Source: CAD feature listing. Evaluate the final solid. Frame: model axes, mm. A direction names the side the tool comes from. Round coordinates to 2 decimals unless told otherwise and drop trailing zeros. Loops run counter-clockwise (first coordinate to the right, second up) from the corner with the lowest first, then second, coordinate; pieces in that order, holes last. Notation, with made-up numbers: M 15,10 L 58,10 A31 ccw 58,41 Z; hole C -12,41 d9. An arc over 180 degrees is marked long. Answer as a JSON object with one key per item and string values.
Autodesk Inventor part; units mm, degrees
ref_plane "YZ Plane" through (0, 0, 0) normal (1, 0, 0) x (0, 1, 0)
ref_plane "XZ Plane" through (0, 0, 0) normal (0, 1, 0) x (-1, 0, 0)
ref_plane "XY Plane" through (0, 0, 0) normal (0, 0, 1) x (1, 0, 0)
sketch "Sketch1" plane through (0, 0, 0) normal (0, 0, 1) x (-1, 0, 0)
  line L0 (0, -67.1677) -> (0, 491.6323)
  line L1 (0, 491.6323) -> (-95.25, 491.6323)
  line L2 (-95.25, 491.6323) -> (-95.25, 485.2823)
  line L3 (-95.25, 485.2823) -> (-63.5, 485.2823)
  line L4 (-63.5, 485.2823) -> (-60.325, 482.1073)
  line L5 (-60.325, 482.1073) -> (-63.5308, 477.5289)
  line L6 (-63.5308, 477.5289) -> (-76.2, 477.5289)
  line L7 (-76.2, 477.5289) -> (-76.2, 375.9289)
  line L8 (-76.2, 375.9289) -> (-133.35, 375.9289)
  line L9 (-133.35, 375.9289) -> (-133.35, 350.5289)
  line L10 (-133.35, 350.5289) -> (-127, 346.0826)
  line L11 (-127, 346.0826) -> (-127, 25.4)
  line L12 (-127, 25.4) -> (-139.7, 25.4)
  line L13 (-139.7, 25.4) -> (-139.7, 0)
  line L14 (-139.7, 0) -> (0, 0)
  line L15 (0, 0) -> (0, 491.6323)
  dimension "d1" = 127
  dimension "d2" = 25.4
  dimension "d3" = 12.7
  dimension "d4" = 95.25
  dimension "d5" = 6.35
  dimension "d6" = 558.8
  dimension "d7" = 6.35
  dimension "d9" = 63.5
  dimension "d10" = 76.2
  dimension "d11" = 101.6
  dimension "d12" = 35
  dimension "d13" = 135
  dimension "d14" = 25.4
  dimension "d15" = 3.175
revolve "Revolution1" add sketch "Sketch1" angle 360 about axis through (0, 67.1677, 0) along (0, -1, 0)
properties part number "Newport SL 1200-422"
Item 1: Section A-A on z = 0. Return the cut outline in (x, y) (3 decimals), then the cut area to 3 significant figures.
Answer sheet:
{"outline": "M -139.7,-25.4 L -127,-25.4 L -127,-346.083 L -133.35,-350.529 L -133.35,-375.929 L -76.2,-375.929 L -76.2,-477.529 L -63.531,-477.529 L -60.325,-482.107 L -63.5,-485.282 L -95.25,-485.282 L -95.25,-491.632 L 95.25,-491.632 L 95.25,-485.282 L 63.5,-485.282 L 60.325,-482.107 L 63.531,-477.529 L 76.2,-477.529 L 76.2,-375.929 L 133.35,-375.929 L 133.35,-350.529 L 127,-346.083 L 127,-25.4 L 139.7,-25.4 L 139.7,0 L -139.7,0 Z", "area": "114,000 mm²"}
Item 2: Pull-direction query (Y, two-part tool) for faces 1 (the flat face through (17, -477.529, -62)), 2 (the flat face through (-2, 0, 2)), 3 (the flat face through (20, -485.282, -62)), 4 (the flat face through (-1, -491.632, 1)); classes: pulls with the +Y half, pulls with the -Y half, needs draft (parallel to the pull), parting line crosses it, or undercut.
Answer sheet:
{"face 1": "undercut", "face 2": "pulls with the +Y half", "face 3": "undercut", "face 4": "pulls with the -Y half"}
Item 3: Access query for faces 5 (the cylindrical face through (-110.86, -12.52, 85.01)), 6 (the cylindrical face through (-75.587, -488.413, 57.958)), 7 (the flat face through (30, -25.4, -124)). Directions: +Z, -Z, +X, -X, +Y, -Y. A direction counts if a zero-diameter tool reaches every point of the face in a straight line with its end or side. Return the directions, or none.
Answer sheet:
{"face 5": "+Y, -Y", "face 6": "-Y", "face 7": "none"}
Item 4: Contact query for flat-ended pins moving along their axis: pin 1 Ø2 at (x, y) = (-14.5, -423.5) entering from +Z; pin 2 Ø5 at (x, y) = (-9, -250.5) entering from -Z; pin 3 Ø10 at (x, y) = (-60, -133) entering from -Z. Output: stop coordinate, or through.
Answer sheet:
{"pin 1": "stops at z = 74.99", "pin 2": "stops at z = -126.83", "pin 3": "stops at z = -114.47"}
Item 5: Line query: probe 1 along Y at (x, z) = (-84, 37.5); probe 2 along Y at (x, z) = (44, -116.5); probe 3 along X at (y, z) = (-422.5, -1). Output: solid intervals per line, ascending. Write a range as from..to.
Answer sheet:
{"probe 1": "y = -491.63..-485.28, -375.93..0", "probe 2": "y = -375.93..0", "probe 3": "x = -76.19..76.19"}
Item 6: Section C-C on x = 0. Return the cut outline in (y, z) (3 decimals), then the cut area to 3 significant figures.
Answer sheet:
{"outline": "M -491.632,-95.25 L -485.282,-95.25 L -485.282,-63.5 L -482.107,-60.325 L -477.529,-63.531 L -477.529,-76.2 L -375.929,-76.2 L -375.929,-133.35 L -350.529,-133.35 L -346.083,-127 L -25.4,-127 L -25.4,-139.7 L 0,-139.7 L 0,139.7 L -25.4,139.7 L -25.4,127 L -346.083,127 L -350.529,133.35 L -375.929,133.35 L -375.929,76.2 L -477.529,76.2 L -477.529,63.531 L -482.107,60.325 L -485.282,63.5 L -485.282,95.25 L -491.632,95.25 Z", "area": "114,000 mm²"}
Item 7: Section B-B on y = -428. Return the cut outline in (x, z), then the cut area to 3 significant figures.
Answer sheet:
{"outline": "C 0,0 d152.4", "area": "18,200 mm²"}
